Geometry: final body of the model. Coordinates: model frame, mm. Face numbers are marked on the shaded views. A direction names the side the tool comes from. Give positions to 0.01 mm unless a question says otherwise; leave off trailing zeros. Write each loop counter-clockwise with the first axis right and the second up, starting at its lowest first coordinate (ties: lowest second). Pieces come first, ordered by that corner, then holes.
from build123d import *

# Parameters (mm, degrees)
EXTRUDE1_DEPTH      = 3.8
EXTRUDE_THIN1_DEPTH = 3.8
SKETCH3_W           = 0.8
SKETCH3_H           = 1.6
CUT_EXTRUDE1_DEPTH  = 0.15
FILLET1_R           = 0.5
SKETCH9_W           = 3.2
SKETCH9_H           = 1.7
SKETCH9_W_2         = 3
SKETCH9_H_2         = 1.5
CUT_EXTRUDE5_DEPTH  = 0.4
SKETCH11_W          = 6
SKETCH11_H          = 3.5
CUT_EXTRUDE6_DEPTH  = 0.01
FILLET6_R           = 0.1
EXTRUDE2_OUTLINE_W  = 2.961598858
EXTRUDE2_OUTLINE_H  = 1.461598858
EXTRUDE2_DEPTH      = 1.5
EXTRUDE2_DRAFT      = 1
FILLET7_R           = 0.2
SKETCH13_W          = 1.27
SKETCH13_H          = 0.4
EXTRUDE3_DEPTH      = 0.4
CUT_EXTRUDE7_DEPTH  = 0.4
CUT_EXTRUDE8_START  = -9.5
CUT_EXTRUDE8_DEPTH  = 2.4
EXTRUDE4_START      = 0.1
EXTRUDE4_DEPTH      = 0.95
SKETCH16_W          = 0.75
SKETCH16_H          = 2
EXTRUDE5_DEPTH      = 0.375
FILLET8_R           = 0.374
EXTRUDE6_DEPTH      = 0.5
EXTRUDE6_DEPTH_BACK = 0.5
EXTRUDE6_START      = -1
SKETCH17_W          = 0.4
SKETCH17_H          = 0.4
FILLET9_R           = 0.5
SKETCH17_3_W        = 0.4
SKETCH17_3_H        = 0.4
EXTRUDE7_DEPTH      = 0.5
EXTRUDE8_DEPTH      = 0.15
EXTRUDE8_DEPTH_BACK = 0.15
EXTRUDE8_START      = -3.5
SKETCH18_W          = 0.5
SKETCH18_H          = 0.15


# Read off the part's stored shape, not the designer's step: Extrude2
with BuildPart() as part:
    # Sketch1 → Extrude1 (new body)
    with BuildSketch(Plane(origin=(0, 0, 0), x_dir=(1, 0, 0), z_dir=(0, 1, 0))):
        Polygon((-1.5, -1.75), (-1.5, -1.45), (1.5, -1.45), (1.5, -1.75), (3, -1.75), (3, 1.75), (-3, 1.75), (-3, -1.75), align=None)
    extrude(amount=EXTRUDE1_DEPTH)

    # Sketch2 → Extrude-Thin1 (add)
    with BuildSketch(Plane(origin=(0, 0, 0), x_dir=(1, 0, 0), z_dir=(0, 1, 0))):
        Polygon((-3.75, -3.95), (-3.75, 2.15), (3.75, 2.15), (3.75, -3.95), (3.35, -3.95), (3.35, 1.75), (-3.35, 1.75), (-3.35, -3.95), align=None)
    extrude(amount=EXTRUDE_THIN1_DEPTH)

    # Sketch3 → Cut-Extrude1 (cut)
    with BuildSketch(Plane(origin=(0, 3.8, 0), x_dir=(-1, 0, 0), z_dir=(0, 1, 0))):
        with Locations((2.6, 0.95)):
            Rectangle(SKETCH3_W, SKETCH3_H)
        with Locations((-2.6, 0.95)):
            Rectangle(SKETCH3_W, SKETCH3_H)
    extrude(amount=-CUT_EXTRUDE1_DEPTH, mode=Mode.SUBTRACT)

    # Fillet1
    fillet1_edges = [part.edges().sort_by_distance(p)[0] for p in [
        (3.55, 3.8, 3.95),
        (3.75, 1.9, -2.15),
        (-3.75, 1.9, -2.15),
        (-3.55, 3.8, 3.95),
    ]]
    fillet(fillet1_edges, radius=FILLET1_R)

    # Sketch9 → Cut-Extrude5 (cut)
    # profile 1 of 2: a face of its own
    with BuildSketch(Plane(origin=(0, 0, -2.15), x_dir=(-1, 0, 0), z_dir=(0, 0, -1))):
        with Locations((0, 1.9)):
            Rectangle(SKETCH9_W, SKETCH9_H)
        with Locations((0, 1.9)):
            Rectangle(SKETCH9_W_2, SKETCH9_H_2, mode=Mode.SUBTRACT)
    # profile 2 of 2: a face of its own
    with BuildSketch(Plane(origin=(0, 0, -2.15), x_dir=(-1, 0, 0), z_dir=(0, 0, -1))):
        with Locations((0, 1.9)):
            Rectangle(SKETCH9_W_2, SKETCH9_H_2)
    extrude(amount=-CUT_EXTRUDE5_DEPTH, mode=Mode.SUBTRACT)

    # Sketch11 → Cut-Extrude6 (cut)
    with BuildSketch(Plane(origin=(0, 3.8, 0), x_dir=(-1, 0, 0), z_dir=(0, 1, 0))):
        Rectangle(SKETCH11_W, SKETCH11_H)
    extrude(amount=-CUT_EXTRUDE6_DEPTH, mode=Mode.SUBTRACT)

    # Fillet6
    fillet6_edges = [part.edges().sort_by_distance(p)[0] for p in [
        (-3.35, 1.9, -1.75),
        (3.35, 1.9, -1.75),
    ]]
    fillet(fillet6_edges, radius=FILLET6_R)


with BuildPart() as extrude2_tool:
    # Extrude2 outline → Extrude2 (with draft: the straight prism first)
    with BuildSketch(Plane(origin=(0, 0, -3.25), x_dir=(-1, 0, 0), z_dir=(0, 0, -1))):
        with Locations((0, 1.9)):
            Rectangle(EXTRUDE2_OUTLINE_W, EXTRUDE2_OUTLINE_H)
    extrude(amount=-EXTRUDE2_DEPTH)
    # Extrude2: the draft: its side faces are tilted about the plane it starts from
    extrude2_sides = [extrude2_tool.faces().sort_by_distance(p)[0] for p in [
        (-1.480799429, 1.9, -2.5),
        (0, 2.630799429, -2.5),
        (1.480799429, 1.9, -2.5),
        (0, 1.169200571, -2.5),
    ]]
    draft(extrude2_sides, Plane(origin=(0, 0, -3.25), x_dir=(-1, 0, 0), z_dir=(0, 0, -1)), EXTRUDE2_DRAFT)


with BuildPart() as part_1:
    add(part.part)

    # Extrude2: add extrude2_tool
    add(extrude2_tool.part)

    # Fillet7
    fillet7_edges = [part_1.edges().sort_by_distance(p)[0] for p in [
        (-1.493890728, 1.156109272, -2.5),
        (-1.480799429, 1.9, -3.25),
        (-1.493890728, 2.643890728, -2.5),
        (0, 2.630799429, -3.25),
        (1.493890728, 2.643890728, -2.5),
        (1.493890728, 1.156109272, -2.5),
        (1.480799429, 1.9, -3.25),
        (0, 1.169200571, -3.25),
    ]]
    fillet(fillet7_edges, radius=FILLET7_R)

    # Sketch13 → Extrude3 (add)
    with BuildSketch(Plane(origin=(0, 0, -2.15), x_dir=(-1, 0, 0), z_dir=(0, 0, -1))):
        with Locations((0, -0.2)):
            Rectangle(SKETCH13_W, SKETCH13_H)
    extrude(amount=-EXTRUDE3_DEPTH)

    # Sketch14 → Cut-Extrude7 (cut)
    with BuildSketch(Plane.ZY.offset(3.75)):
        Polygon((-0.475, 1.325), (0.45, 1.325), (1.375, 1.325), (1.375, 2.475), (-0.475, 2.475), align=None)
        Polygon((0.2, 0.15), (0.1, 0), (0.8, 0), (0.7, 0.15), align=None)
    extrude(amount=-CUT_EXTRUDE7_DEPTH, mode=Mode.SUBTRACT)

    # Sketch14<3> → Cut-Extrude8 (cut)
    with BuildSketch(Plane.ZY.offset(3.75).offset(CUT_EXTRUDE8_START)):
        Polygon((-0.475, 1.325), (0.45, 1.325), (1.375, 1.325), (1.375, 2.475), (-0.475, 2.475), align=None)
        Polygon((0.2, 0.15), (0.1, 0), (0.8, 0), (0.7, 0.15), align=None)
    extrude(amount=CUT_EXTRUDE8_DEPTH, mode=Mode.SUBTRACT)

    # Sketch15 → Extrude4 (add)
    with BuildSketch(Plane(origin=(0, 1.325, 0), x_dir=(-1, 0, 0), z_dir=(0, 1, 0)).offset(EXTRUDE4_START)):
        Polygon((3, 1.375), (3.65, 1.375), (3.65, 0.175), (3, -0.625), align=None)
        Polygon((-3, -0.625), (-3, 1.375), (-3.65, 1.375), (-3.65, 0.175), align=None)
    extrude(amount=EXTRUDE4_DEPTH)

    # Sketch16 → Extrude5 (add)
    with BuildSketch(Plane(origin=(0, 0, -2.15), x_dir=(-1, 0, 0), z_dir=(0, 0, -1))):
        with Locations((-2.625, 1.9)):
            Rectangle(SKETCH16_W, SKETCH16_H)
        with Locations((2.625, 1.9)):
            Rectangle(SKETCH16_W, SKETCH16_H)
    extrude(amount=EXTRUDE5_DEPTH)

    # Fillet8
    fillet8_edges = [part_1.edges().sort_by_distance(p)[0] for p in [
        (3, 2.9, -2.3375),
        (3, 0.9, -2.3375),
        (2.25, 0.9, -2.3375),
        (2.25, 2.9, -2.3375),
        (3, 1.9, -2.525),
        (2.625, 0.9, -2.525),
        (2.25, 1.9, -2.525),
        (2.625, 2.9, -2.525),
        (-3, 2.9, -2.3375),
        (-2.25, 2.9, -2.3375),
        (-2.25, 0.9, -2.3375),
        (-3, 0.9, -2.3375),
        (-2.625, 2.9, -2.525),
        (-2.25, 1.9, -2.525),
        (-2.625, 0.9, -2.525),
        (-3, 1.9, -2.525),
    ]]
    fillet(fillet8_edges, radius=FILLET8_R)

    # Sketch17 → Extrude6 (add, two sides: drawn at the far end of the back side and taken through both)
    with BuildSketch(Plane.XY.offset(3.95).offset(EXTRUDE6_START - EXTRUDE6_DEPTH_BACK)):
        Polygon((-3.35, -0.4), (-3.75, -0.4), (-3.75, -0.9), (-4.25, -2.1), (-3.7, -3.1), (-3.7, -3.6), (-3.5, -3.6), (-3.3, -3.6), (-3.3, -2.997257294), (-3.806677376, -2.076025702), (-3.35, -0.98), align=None)
        with Locations((-3.55, -0.2)):
            Rectangle(SKETCH17_W, SKETCH17_H)
        with Locations((3.55, -0.2)):
            Rectangle(SKETCH17_W, SKETCH17_H)
        Polygon((3.75, -0.4), (3.35, -0.4), (3.35, -0.98), (3.806677376, -2.076025702), (3.3, -2.997257294), (3.3, -3.6), (3.5, -3.6), (3.7, -3.6), (3.7, -3.1), (4.25, -2.1), (3.75, -0.9), align=None)
    extrude(amount=EXTRUDE6_DEPTH + EXTRUDE6_DEPTH_BACK)

    # Fillet9
    fillet9_edges = [part_1.edges().sort_by_distance(p)[0] for p in [
        (3.5, -3.6, 3.45),
        (3.5, -3.6, 2.45),
        (-3.5, -3.6, 3.45),
        (-3.5, -3.6, 2.45),
    ]]
    fillet(fillet9_edges, radius=FILLET9_R - 0.0001)  # a hair under: the kernel refuses the full size

    # Sketch17<3> → Extrude7 (add)
    with BuildSketch(Plane.XY.offset(3.95)):
        with Locations((-3.55, -0.2)):
            Rectangle(SKETCH17_3_W, SKETCH17_3_H)
        with Locations((3.55, -0.2)):
            Rectangle(SKETCH17_3_W, SKETCH17_3_H)
    extrude(amount=-EXTRUDE7_DEPTH)

    # Sketch18 → Extrude8 (add, two sides: drawn at the far end of the back side and taken through both)
    with BuildSketch(Plane.XY.offset(3.95).offset(EXTRUDE8_START - EXTRUDE8_DEPTH_BACK)):
        Polygon((2.75, 0), (2.25, 0), (2.25, -3), (2.5, -3), (2.75, -3), align=None)
        Polygon((-2.5, -3), (-2.25, -3), (-2.25, 0), (-2.75, 0), (-2.75, -3), align=None)
        with Locations((-2.5, 3.725)):
            Rectangle(SKETCH18_W, SKETCH18_H)
        with Locations((2.5, 3.725)):
            Rectangle(SKETCH18_W, SKETCH18_H)
    extrude(amount=EXTRUDE8_DEPTH + EXTRUDE8_DEPTH_BACK)


solid = part_1.part
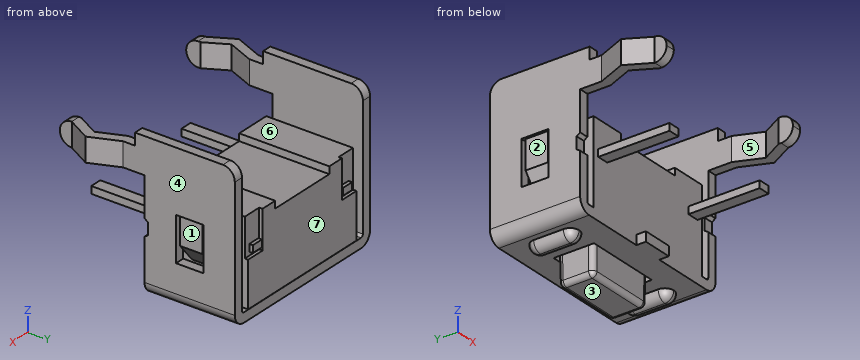
Q1. Pull-direction query (Z, two-part tool) for the marked faces 1, 2, 3 and 4; classes: released by +Z, released by -Z, zero draft, split by the parting line, or undercut.
Filled sheet:
face 1: undercut
face 2: undercut
face 3: released by -Z
face 4: zero draft
Q2. Ray query, line 1 along X through (y, z) = (0.25, 1.5); line 2 along X through (y, z) = (2.75, 1); line 3 along X through (y, z) = (-0.5, 0.5). Return the intervals inside material, ascending.
Filled sheet:
line 1: x = -3.75 to -3.35, -3 to -1.5, 1.5 to 3, 3.35 to 3.75
line 2: x = -3.75 to -3.35, -3 to 3, 3.35 to 3.75
line 3: x = -2.75 to -2.25, 2.25 to 2.75
Q3. Section D-D on y = 0.75. Output: boundary loops of the cut face in (x, z).
Filled sheet:
outline: (-3.75, -1.65) arc R0.5 ccw to (-3.25, -2.15) - (3.25, -2.15) arc R0.5 ccw to (3.75, -1.65) - (3.75, 3.95) - (3.35, 3.95) - (3.35, -1.65) arc R0.1 cw to (3.25, -1.75) - (3, -1.75) - (3, 1.75) - (1.5, 1.75) - (1.5, 1.45) - (-1.5, 1.45) - (-1.5, 1.75) - (-3, 1.75) - (-3, -1.75) - (-3.25, -1.75) arc R0.1 cw to (-3.35, -1.65) - (-3.35, 3.95) - (-3.75, 3.95) - close
Q4. Access query for the marked faces 5, 6 and 7. Directions: +Z, -Z, +X, -X, +Y, -Y. A direction counts if a zero-diameter tool reaches every point of the face in a straight line with its end or side. Return the directions, or none.
Filled sheet:
face 5: +Z, -Z
face 6: +Z, +Y, -Y
face 7: +Y
Q5. Section B-B on z = -0.25. Output: boundary loops of the cut face in (x, y) (3 decimals), plus the area to 3 significant figures.
Filled sheet:
outline: (-3.75, 0) - (-3.35, 0) - (-3.35, 1.325) - (-3.75, 1.325) - close; (-3.75, 2.475) - (-3.35, 2.475) - (-3.35, 3.8) - (-3.75, 3.8) - close; (-3.305, 1.425) - (-3, 1.425) - (-3, 0) - (3, 0) - (3, 1.425) - (3.305, 1.425) - (3.305, 2.375) - (3, 2.375) - (3, 3.79) - (-3, 3.79) - (-3, 2.375) - (-3.305, 2.375) - close; (3.35, 0) - (3.75, 0) - (3.75, 1.325) - (3.35, 1.325) - close; (3.35, 2.475) - (3.75, 2.475) - (3.75, 3.8) - (3.35, 3.8) - close
area: 25.4 mm2
Q6. Section A-A on y = -2.5. Output: boundary loops of the cut face in (x, z), plus the area to 3 significant figures.
Filled sheet:
outline: (-4.03, 2.45) - (-3.57, 2.45) - (-3.57, 3.45) - (-4.03, 3.45) - close; (-2.75, 0.3) - (-2.25, 0.3) - (-2.25, 0.6) - (-2.75, 0.6) - close; (2.25, 0.3) - (2.75, 0.3) - (2.75, 0.6) - (2.25, 0.6) - close; (3.57, 2.45) - (4.03, 2.45) - (4.03, 3.45) - (3.57, 3.45) - close
area: 1.21 mm2
Q7. Pin query (flat end, axial travel): P1, Ø1, axis at y = 1.5, z = 1.5, coming from the +X side; P2, Ø3, axis at x = 1, z = 1.5, coming from the +Y side; P3, Ø4, axis at y = 0.5, z = 2.5, coming from the -X side. Return the tip coordinate at first contact, or that it passes through.
Filled sheet:
P1: stops at x = 3.75
P2: stops at y = 3.79
P3: stops at x = -4
